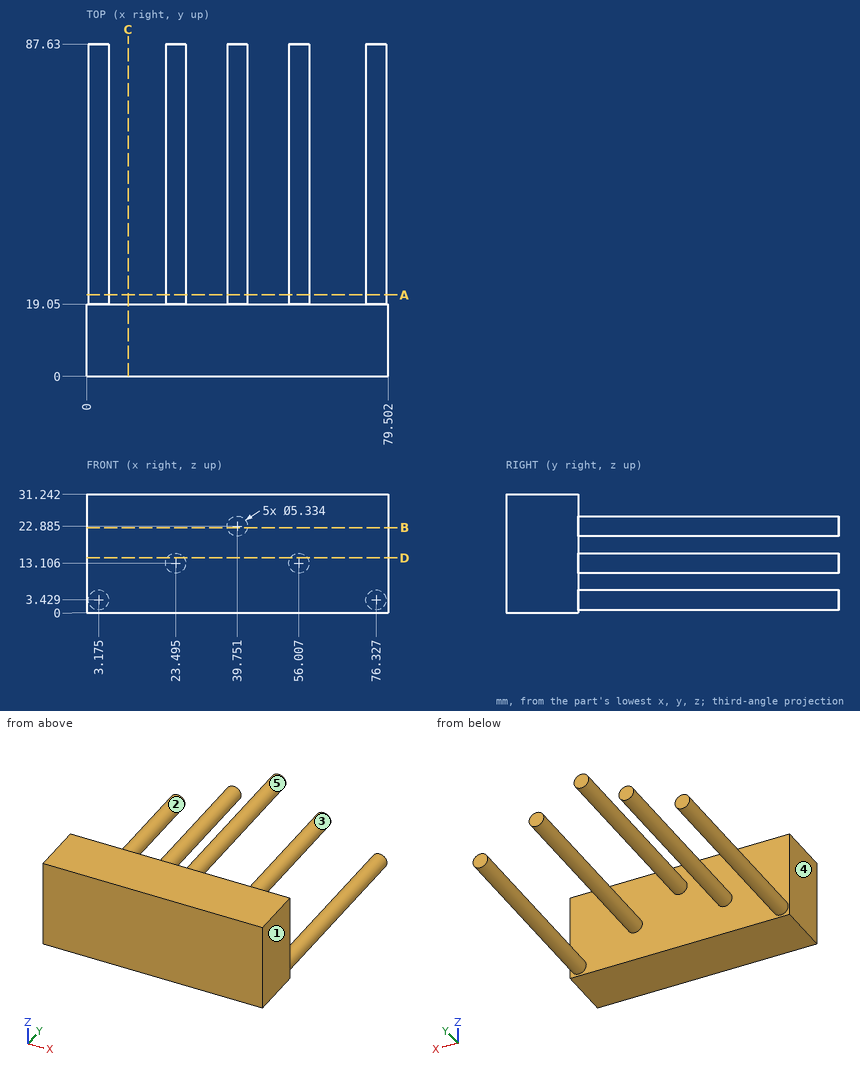
Answer from the drawing. Dimensions are ordinates in mm from the lowest x, y and z of the part. A direction names the side the tool comes from. Round coordinates to 2 decimals unless told otherwise and drop trailing zeros. Order: outer loops, then holes, each group sorted by start corner. A loop starts at its lowest first (then second) coordinate and runs counter-clockwise, first axis right, second up.
1) The mould has two halves that part along X. Classify the marked faces 3, 4 and 5: released by +X, released by -X, zero draft, split by the parting line, or undercut.
2) The part is cut by section A-A on y = 21.5. Write down the section's boundary in (x, z) (3 decimals), plus the area to 3 significant figures.
3) Straight lines are drawn through the part: L1, parallel to Y at x = 71, z = 18; L2, parallel to X at y = 66.5, z = 2.5 (1 decimal); L3, parallel to X at y = 58, z = 23. For each, find the intervals that lie inside material, in ascending order.
4) The part is cut by section D-D on z = 14.5. Write down the section's boundary in (x, y).
5) The part is cut by section B-B on z = 22.5. Write down the section's boundary in (x, y).
6) Flat-ended cylindrical pins translate along their axes: pin 1 (5 mm diameter, centred on y = 55, z = 11.5, fed in from +X); pin 2 (3 mm diameter, centred on y = 58.5, z = 21, fed in from +X); pin 3 (4 mm diameter, centred on x = 28.5, y = 61.5, fed in from -Z); pin 4 (4 mm diameter, centred on x = 47.5, z = 4.5, fed in from +Y). Find the tip coordinate at first contact, or state that the pin passes through.
7) For the marked faces 1 and 2, determine the directions among +Z, -Z, +X, -X, +Y, -Y from which every point of the face is accessible in a straight line to the end or side of a thin tool.
8) The part is cut by section C-C on x = 11. Write down the section's boundary in (y, z), plus the area to 3 significant figures.
Resolved:
1. face 3: undercut
1. face 4: released by -X
1. face 5: split by the parting line
2. outline: circle Ø5.334 at (3.175, 3.429); circle Ø5.334 at (23.495, 13.106); circle Ø5.334 at (39.751, 22.885); circle Ø5.334 at (56.007, 13.106); circle Ø5.334 at (76.327, 3.429)
2. area: 112 mm2
3. L1: y = 0 to 19.05
3. L2: x = 0.7 to 5.7, 73.8 to 78.8
3. L3: x = 37.09 to 42.42
4. outline: (0, 0) - (79.5, 0) - (79.5, 19.05) - (58.28, 19.05) - (58.28, 87.63) - (53.73, 87.63) - (53.73, 19.05) - (25.77, 19.05) - (25.77, 87.63) - (21.22, 87.63) - (21.22, 19.05) - (0, 19.05) - close
5. outline: (0, 0) - (79.5, 0) - (79.5, 19.05) - (42.39, 19.05) - (42.39, 87.63) - (37.11, 87.63) - (37.11, 19.05) - (0, 19.05) - close
6. pin 1: stops at x = 58.67
6. pin 2: stops at x = 42.39
6. pin 3: passes through
6. pin 4: stops at y = 19.05
7. face 1: +Z, -Z, +X, +Y, -Y
7. face 2: +Y
8. outline: (0, 0) - (19.05, 0) - (19.05, 31.24) - (0, 31.24) - close
8. area: 595 mm2
